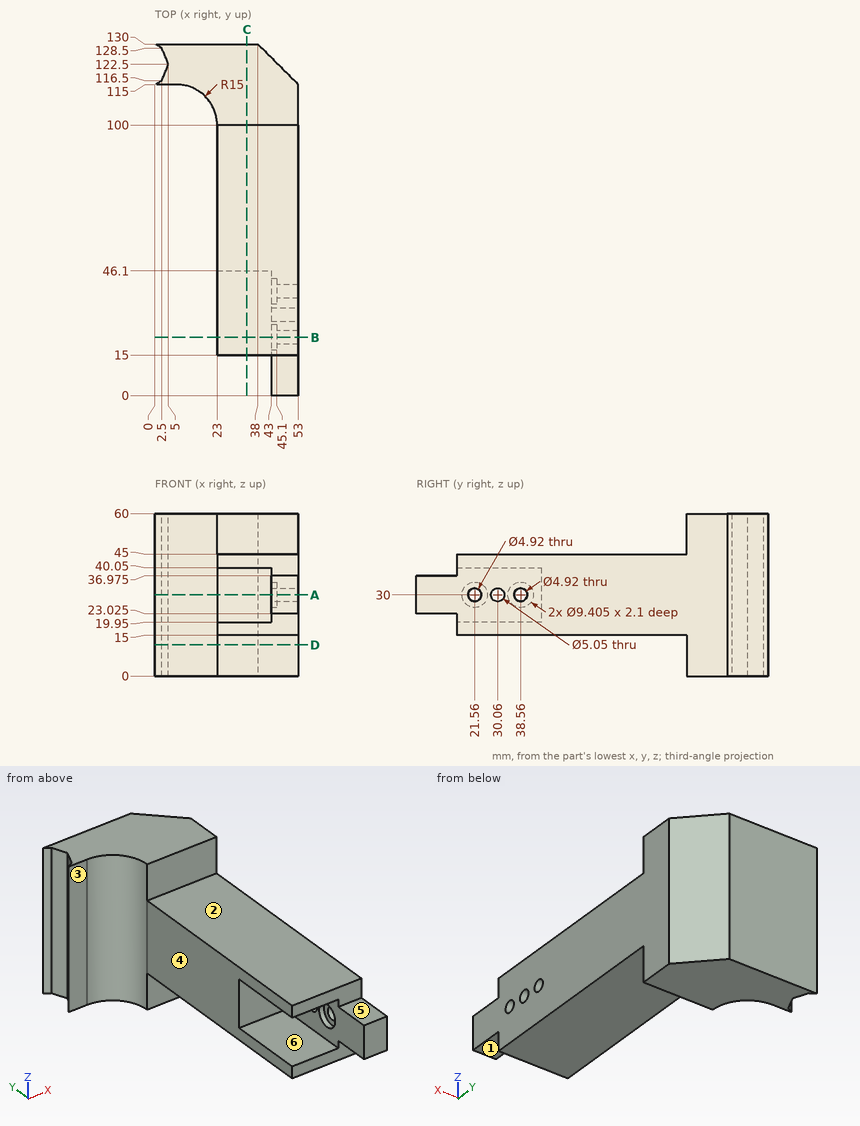
Check sheet for the drawn part. Datum: minimum x, y, z corner. Units: mm. A direction names the side the tool comes from. Round coordinates to 2 decimals unless told otherwise and drop trailing zeros. Order: outer loops, then holes, each group sorted by start corner. A loop starts at its lowest first (then second) coordinate and runs counter-clockwise, first axis right, second up. Notation, with made-up numbers: (88, 40.25) -> (125, 40.25) arc R23 ccw to (125, 50.25) -> close; hole circle Ø2 at (73, -27). An arc over 180 degrees is marked (long way). Put each result on its own line as item: value.
1) Section check A-A (z = 30). Give the number of separate pieces and of enclosed holes in the cut face, then the cut area to 3 significant figures.
Final values:
separate pieces: 4
enclosed holes: 0
area: 3,040 mm^2
2) Mould release check, pull along Z, two halves, no side actions. Record for the marked faces 4, 5 and 6: +Z half, -Z half, draft (parallel to the pull), parting line (faces both ways), or undercut.
Final values:
face 4: draft
face 5: +Z half
face 6: undercut
3) Section check C-C (x = 34). Record the cut outline in (y, z).
Final values:
outline: (15, 15) -> (100, 15) -> (100, 0) -> (130, 0) -> (130, 60) -> (100, 60) -> (100, 45) -> (15, 45) -> (15, 40.05) -> (46.1, 40.05) -> (46.1, 19.95) -> (15, 19.95) -> close
4) Section check D-D (z = 11.5). Record the cut outline in (x, y).
Final values:
outline: (0, 115) -> (8, 115) arc R15 cw to (23, 100) -> (53, 100) -> (53, 115) -> (38, 130) -> (0, 130) -> (2.5, 128.5) -> (5, 122.5) -> (2.5, 116.5) -> close
5) Section check B-B (y = 21.56). Record the cut outline in (x, z), then the cut area to 3 significant figures.
Final values:
outline: (23, 15) -> (53, 15) -> (53, 27.54) -> (45.1, 27.54) -> (45.1, 25.3) -> (43, 25.3) -> (43, 19.95) -> (23, 19.95) -> close; (23, 40.05) -> (43, 40.05) -> (43, 34.7) -> (45.1, 34.7) -> (45.1, 32.46) -> (53, 32.46) -> (53, 45) -> (23, 45) -> close
area: 439 mm^2
6) Material ranges on line 1 (Z direction, x = 50, y = 21.56); line 2 (Z direction, x = 31, y = 56); line 3 (Y direction, x = 6.5, z = 7), recorded low to high.
Final values:
line 1: z = 15 to 27.54, 32.46 to 45
line 2: z = 15 to 45
line 3: y = 115 to 130
7) Set-up check for the marked faces 1, 2 and 3: record each of +Z, -Z, +X, -X, +Y, -Y from which the full face is reachable in a straight line by a thin tool's end or side.
Final values:
face 1: -Z, +X, -X, -Y
face 2: +Z, +X, -X, -Y
face 3: +Z, -Z, -X, -Y
8) Depth check by flat-ended pin: pin 1 (10 mm diameter, centred on x = 30.5, z = 33, fed in from -Y); pin 2 (1.5 mm diameter, centred on x = 42, y = 83, fed in from +Z); pin 3 (6 mm diameter, centred on x = 33.5, y = 33.5, fed in from -Z); pin 4 (8.5 mm diameter, centred on y = 38.56, z = 30, fed in from +X). Enter the tip coordinate at first touch or a pass-through.
Final values:
pin 1: stops at y = 46.1
pin 2: stops at z = 45
pin 3: stops at z = 15
pin 4: stops at x = 53
